from build123d import *
from build123d.topology import SkipClean

# Parameters (mm, degrees)
SKETCH1_R                      = 12.3
SKETCH1_R_2                    = 11.45
SKETCH1_R_3                    = 9
SKETCH1_R_4                    = 8.15
BOSS_EXTRUDE4_DEPTH            = 59
SKETCH1_8_R                    = 5
BOSS_EXTRUDE17_DEPTH           = 10
BOSS_EXTRUDE17_DRAFT           = 1
BOSS_EXTRUDE17_PROFILE_2_DEPTH = 10
BOSS_EXTRUDE17_PROFILE_2_DRAFT = 1
BOSS_EXTRUDE19_DEPTH           = 59
SKETCH17_R                     = 11.45
SKETCH17_R_2                   = 8.15
BOSS_EXTRUDE20_DEPTH           = 3
SKETCH19_R                     = 3.2
CUT_EXTRUDE5_DEPTH             = 10
BOSS_EXTRUDE21_DEPTH           = 10
CUT_EXTRUDE8_DEPTH             = 66
CUT_EXTRUDE9_DEPTH             = 2
BOSS_EXTRUDE24_DEPTH           = 3.5
FILLET1_R                      = 2
FILLET2_R                      = 0.5


with BuildPart() as part:
    # Sketch1 → Boss-Extrude4 (new body)
    # profile 1 of 2: a face of its own
    with BuildSketch(Plane(origin=(0, 0, 0), x_dir=(1, 0, 0), z_dir=(0, 1, 0))):
        with Locations((35.202950653, 27.384819692)):
            Circle(SKETCH1_R)
        with Locations(Location((35.202950653, 27.384819692, 0), (0, 0, 270))):
            Circle(SKETCH1_R_2, mode=Mode.SUBTRACT)
    # profile 2 of 2: a face of its own
    with BuildSketch(Plane(origin=(0, 0, 0), x_dir=(1, 0, 0), z_dir=(0, 1, 0))):
        with Locations((22.493671705, 43.629178782)):
            Circle(SKETCH1_R_3)
        with Locations(Location((22.493671705, 43.629178782, 0), (0, 0, 270))):
            Circle(SKETCH1_R_4, mode=Mode.SUBTRACT)
    extrude(amount=BOSS_EXTRUDE4_DEPTH)

    # Sketch12 → Boss-Extrude19 (add)
    with SkipClean():  # the faces are left unmerged after this step: merging them gives an invalid solid
        with BuildSketch(Plane(origin=(0, 0, 0), x_dir=(-1, 0, 0), z_dir=(0, -1, 0))):
            with BuildLine():
                Line((-34.977539895, 38.8326007), (-30.605091655, 44.421243424))
                ThreePointArc((-30.605091655, 44.421243424), (-27.821958355, 37.462181021), (-20.532623065, 35.718629608))
                Line((-20.532623065, 35.718629608), (-24.304935413, 30.897050301))
                ThreePointArc((-24.304935413, 30.897050301), (-28.370974986, 36.573215009), (-34.977539895, 38.8326007))
            make_face()
        extrude(amount=-BOSS_EXTRUDE19_DEPTH)



with BuildPart() as body_2:
    # Sketch1<8> → Boss-Extrude17 (with draft: the straight prism first)
    with BuildSketch(Plane(origin=(0, 0, 0), x_dir=(1, 0, 0), z_dir=(0, 1, 0))):
        with Locations((22.493671705, 43.629178782)):
            Circle(SKETCH1_8_R)
    extrude(amount=BOSS_EXTRUDE17_DEPTH)
    # Boss-Extrude17: the draft: its side faces are tilted about the plane it starts from
    boss_extrude17_sides = [body_2.faces().sort_by_distance(p)[0] for p in [
        (17.493671705, 5, -43.629178782),
    ]]
    draft(boss_extrude17_sides, Plane(origin=(0, 0, 0), x_dir=(1, 0, 0), z_dir=(0, 1, 0)), BOSS_EXTRUDE17_DRAFT)


with BuildPart() as body_3:
    # Sketch1<8> → Boss-Extrude17 profile 2 (with draft: the straight prism first)
    with BuildSketch(Plane(origin=(0, 0, 0), x_dir=(1, 0, 0), z_dir=(0, 1, 0))):
        with Locations((35.202950653, 27.384819692)):
            Circle(SKETCH1_8_R)
    extrude(amount=BOSS_EXTRUDE17_PROFILE_2_DEPTH)
    # Boss-Extrude17 profile 2: the draft: its side faces are tilted about the plane it starts from
    boss_extrude17_profile_2_sides = [body_3.faces().sort_by_distance(p)[0] for p in [
        (30.202950653, 5, -27.384819692),
    ]]
    draft(boss_extrude17_profile_2_sides, Plane(origin=(0, 0, 0), x_dir=(1, 0, 0), z_dir=(0, 1, 0)), BOSS_EXTRUDE17_PROFILE_2_DRAFT)


with BuildPart() as part_1:
    with SkipClean():  # the faces are left unmerged after this step: merging them gives an invalid solid
        add(part.part)

        add(body_2.part)  # Boss-Extrude20 merges body 2

        add(body_3.part)  # Boss-Extrude20 merges body 3
        # Sketch17 → Boss-Extrude20 (add)
        with BuildSketch(Plane.XZ):
            with Locations(Location((35.202950653, -27.384819692, 0), (0, 0, 270))):
                Circle(SKETCH17_R)
            with Locations(Location((22.493671705, -43.629178782, 0), (0, 0, 270))):
                Circle(SKETCH17_R_2)
        extrude(amount=-BOSS_EXTRUDE20_DEPTH)

    # Sketch19 → Cut-Extrude5 (cut)
    with SkipClean():  # the faces are left unmerged after this step: merging them gives an invalid solid
        with BuildSketch(Plane(origin=(0, 0, 0), x_dir=(-1, 0, 0), z_dir=(0, -1, 0))):
            with Locations(Location((-35.202950653, 27.384819692, 0), (0, 0, 90))):
                Circle(SKETCH19_R)
            with Locations(Location((-22.493671705, 43.629178782, 0), (0, 0, 90))):
                Circle(SKETCH19_R)
        extrude(amount=-CUT_EXTRUDE5_DEPTH, mode=Mode.SUBTRACT)

    # Sketch35 → Cut-Extrude8 (cut)
    with BuildSketch(Plane.XZ):
        with BuildLine():
            Line((21.325413706, -34.705324611), (23.682144413, -31.693070334))
            ThreePointArc((23.682144413, -31.693070334), (42.566125739, -17.532223454), (34.334781161, -39.654142483))
            Line((34.334781161, -39.654142483), (31.487409842, -43.293508835))
            ThreePointArc((31.487409842, -43.293508835), (16.684303244, -50.503132381), (21.325413706, -34.705324611))
        make_face()
    extrude(amount=-CUT_EXTRUDE8_DEPTH, mode=Mode.SUBTRACT)


with BuildPart() as body_2_2:
    # Sketch23 → Boss-Extrude21 (new body)
    with BuildSketch(Plane(origin=(0, 59, 0), x_dir=(1, 0, 0), z_dir=(0, 1, 0))):
        with BuildLine():
            Line((37.468337272, 40.662183298), (32.546981676, 46.25595936))
            ThreePointArc((32.546981676, 46.25595936), (15.596937819, 51.401184911), (18.690039782, 33.959566495))
            Line((18.690039782, 33.959566495), (21.882803933, 29.3833322))
            ThreePointArc((21.882803933, 29.3833322), (43.099472085, 16.473114504), (37.468337272, 40.662183298))
        make_face()
        with BuildLine():
            ThreePointArc((21.325413706, 34.705324611), (16.684303244, 50.503132381), (31.487409842, 43.293508835))
            Line((31.487409842, 43.293508835), (34.334781161, 39.654142483))
            ThreePointArc((34.334781161, 39.654142483), (42.566125739, 17.532223454), (23.682144413, 31.693070334))
            Line((23.682144413, 31.693070334), (21.325413706, 34.705324611))
        make_face(mode=Mode.SUBTRACT)
    extrude(amount=BOSS_EXTRUDE21_DEPTH)

    # Sketch36 → Cut-Extrude9 (cut)
    with BuildSketch(Plane(origin=(0, 69, 0), x_dir=(1, 0, 0), z_dir=(0, 1, 0))):
        with BuildLine():
            Line((43.099472085, 16.473114504), (16.167051125, 51.87192648))
            ThreePointArc((16.167051125, 51.87192648), (12.204421781, 42.179919116), (18.690039782, 33.959566495))
            Line((18.690039782, 33.959566495), (21.882803933, 29.3833322))
            ThreePointArc((21.882803933, 29.3833322), (28.201353831, 15.878386587), (43.099472085, 16.473114504))
        make_face()
    extrude(amount=-CUT_EXTRUDE9_DEPTH, mode=Mode.SUBTRACT)

    # Sketch37 → Boss-Extrude24 (add)
    with BuildSketch(Plane(origin=(0, 69, 0), x_dir=(1, 0, 0), z_dir=(0, 1, 0))):
        with BuildLine():
            ThreePointArc((34.334781161, 39.654142483), (46.768156488, 31.572422107), (42.391274941, 17.403938272))
            Line((42.391274941, 17.403938272), (43.099472085, 16.473114504))
            ThreePointArc((43.099472085, 16.473114504), (48.321405443, 30.438752363), (37.468337272, 40.662183298))
            Line((37.468337272, 40.662183298), (32.546981676, 46.25595936))
            ThreePointArc((32.546981676, 46.25595936), (25.863660596, 53.45832892), (16.167051125, 51.87192648))
            Line((16.167051125, 51.87192648), (17.009199279, 50.765043285))
            ThreePointArc((17.009199279, 50.765043285), (26.620982357, 51.627010161), (31.487409842, 43.293508835))
            Line((31.487409842, 43.293508835), (34.334781161, 39.654142483))
        make_face()
        with BuildLine():
            Line((40.265515658, 20.197944547), (42.391274941, 17.403938272))
            ThreePointArc((42.391274941, 17.403938272), (46.768156488, 31.572422107), (34.334781161, 39.654142483))
            Line((34.334781161, 39.654142483), (31.487409842, 43.293508835))
            ThreePointArc((31.487409842, 43.293508835), (26.620982357, 51.627010161), (17.009199279, 50.765043285))
            Line((17.009199279, 50.765043285), (18.297152058, 49.072213728))
            ThreePointArc((18.297152058, 49.072213728), (25.526405421, 49.79683091), (29.366619149, 43.629178782))
            ThreePointArc((29.366619149, 43.629178782), (28.641776112, 40.557010367), (26.620135535, 38.132843382))
            Line((26.620135535, 38.132843382), (29.626833273, 34.180969615))
            ThreePointArc((29.626833273, 34.180969615), (38.962032304, 35.331519884), (43.993897063, 27.384819692))
            ThreePointArc((43.993897063, 27.384819692), (43.006330576, 23.336610142), (40.265515658, 20.197944547))
        make_face()
    extrude(amount=BOSS_EXTRUDE24_DEPTH)

    # Fillet1
    fillet1_edges = [body_2_2.edges().sort_by_distance(p)[0] for p in [
        (29.626833273, 70.75, -34.180969615),
        (40.265515658, 70.75, -20.197944547),
        (18.297152058, 70.75, -49.072213728),
        (26.620135535, 70.75, -38.132843382),
    ]]
    fillet(fillet1_edges, radius=FILLET1_R)

    # Fillet2
    fillet2_edges = [body_2_2.edges().sort_by_distance(p)[0] for p in [
        (42.199176887, 72.5, -32.707747202),
        (27.963469036, 72.5, -47.790755853),
        (28.095359601, 72.5, -36.193872526),
        (18.322601236, 72.5, -49.761580581),
        (27.291314439, 72.5, -37.973490947),
        (29.660488695, 72.5, -34.92920458),
        (40.995618754, 72.5, -20.030798741),
        (48.321405443, 72.5, -30.438752363),
        (35.007659474, 72.5, -43.459071329),
        (25.863660596, 72.5, -53.45832892),
        (16.692641456, 72.5, -51.181113228),
        (42.25007881, 72.5, -17.589520374),
    ]]
    fillet(fillet2_edges, radius=FILLET2_R)


solid = body_2_2.part
Model file for the job. Use its own axes, mm. A direction names the side the tool comes from. Round coordinates to 2 decimals unless told otherwise and drop trailing zeros. Order: outer loops, then holes, each group sorted by start corner. A loop starts at its lowest first (then second) coordinate and runs counter-clockwise, first axis right, second up.
(1) 3-axis set-ups, long thin cutter, end or side, ignore diameter. For faces 1 (the face through (23, 67, -30)), 2 (the face through (22.52, 62.94, -33.18)), 3 (the face through (20.52, 63.93, -52.41)): which of +Z, -Z, +X, -X, +Y, -Y reach the whole face in a straight line?
(2) Pin check, flat tips, straight feed: pin 1 (3 mm diameter, centred on x = 26.5, z = -36.5, fed in from -Y); pin 2 (1.5 mm diameter, centred on y = 69, z = -39.5, fed in from -X); pin 3 (3 mm diameter, centred on x = 18, y = 68.5, fed in from -Z). Stop position of each tip, or through.
(3) Pull direction X, two halves, no side cores. Call faces 4 (the face through (28.22, 72.36, -36.28)), 5 (the face through (32.89, 63.93, -41.5)), 6 (the face through (34.878, 72.357, -43.378)): released by +X, released by -X, zero draft, split by the parting line, or undercut.
(4) Band-saw the part on A-A (y = 62). List the corners of the cut face in (x, z), then the cut area to 3 significant figures.
(5) Band-saw the part on B-B (y = 67.5). List the corners of the cut face in (x, z), then the cut area to 3 significant figures.
(6) Drill centre lines: line 1 (Z direction, x = 26.5, y = 66.5); line 2 (Z direction, x = 26, y = 63.5); line 3 (Y direction, x = 16.5, z = -36). Where is each one in solid material? Low to high.
Verdict:
1. face 1: +Z, -X, +Y
1. face 2: +Y, -Y
1. face 3: -Y
2. pin 1: stops at y = 69
2. pin 2: stops at x = 27.47
2. pin 3: stops at z = -53.58
3. face 4: released by -X
3. face 5: undercut
3. face 6: released by +X
4. outline: (18.69, -33.96) arc R10.39 ccw (long way) to (32.55, -46.26) - (37.47, -40.66) arc R13.47 ccw (long way) to (21.88, -29.38) - close; hole (21.33, -34.71) arc R9 ccw (long way) to (31.49, -43.29) - (34.33, -39.65) arc R12.3 ccw (long way) to (23.68, -31.69) - close
4. area: 162 mm2
5. outline: (16.17, -51.87) arc R10.39 ccw to (32.55, -46.26) - (37.47, -40.66) arc R13.47 ccw to (43.1, -16.47) - (42.39, -17.4) arc R12.3 cw to (34.33, -39.65) - (31.49, -43.29) arc R9 cw to (17.01, -50.77) - close
5. area: 82.5 mm2
6. line 1: z = -53.22 to -51.69, -18.69 to -17.1
6. line 2: z = -53.41 to -51.92, -19.22 to -17.55
6. line 3: y = 59 to 67
